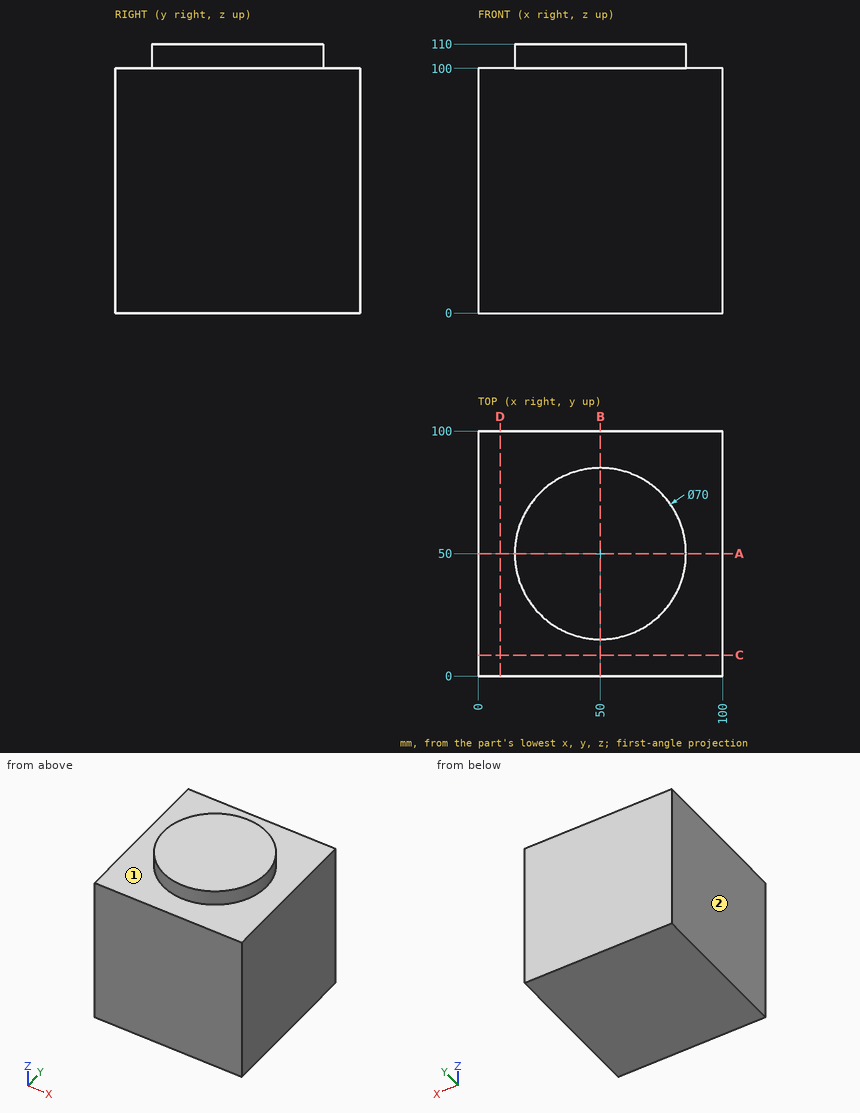
Geometry: see drawing. Coordinates: mm, zero at the bounding-box minimum. A direction names the side the tool comes from. Round coordinates to 2 decimals unless told otherwise and drop trailing zeros. Write each loop counter-clockwise with the first axis right and the second up, starting at its lowest first coordinate (ties: lowest second). Pieces come first, ordered by that corner, then holes. Notation, with made-up numbers: (-22, 73.25) - (0, 73.25) arc R21 ccw to (0, 109.25) - close; hole circle Ø3 at (46, -22). An arc over 180 degrees is marked (long way). Use CSV: the item, a comma, the result in double quotes. Start each with the question number.
(1) Cut plane C-C, the plane y = 8.5. Return loops of the section in (x, z), and give its area (3 significant figures).
(2) Set-up query: the marked faces 1 and 2. Return all of +Z, -Z, +X, -X, +Y, -Y with unobstructed straight access to the full face (end or side cutting, diameter ignored); none if empty.
(3) First-contact query: pin 1 Ø12 at (x, y) = (65, 82.5) entering from -Z; pin 2 Ø8 at (x, y) = (16.5, 26.5) entering from +Z. Flat tips, straight axial feed; report the tip coordinate or a pass-through.
(4) Cut plane A-A, the plane y = 50. Return loops of the section in (x, z).
(5) Material intervals for probe 1 along Z at (x, y) = (12, 88), sorted ascending. Write a range as [from, to].
Geometry says:
1,outline,"(0, 0) - (100, 0) - (100, 100) - (0, 100) - close"
1,area,"10,000 mm²"
2,face 1,"+Z"
2,face 2,"+Z, -Z, -X, +Y, -Y"
3,pin 1,"z = 0"
3,pin 2,"z = 100"
4,outline,"(0, 0) - (100, 0) - (100, 100) - (85, 100) - (85, 110) - (15, 110) - (15, 100) - (0, 100) - close"
5,probe 1,"[0, 100]"
